Geometry check sheet. Reference: the model listing, model coordinates, mm. Face numbers are marked on the shaded views. A direction names the side the tool comes from. Coordinates: 2 decimals unless noted, no trailing zeros. Write each loop counter-clockwise with the first axis right and the second up, starting at its lowest first coordinate (ties: lowest second). Pieces come first, ordered by that corner, then holes. Notation, with made-up numbers: (-6.75, -15.75) -> (43.25, -15.75) arc R30 ccw to (43.25, 11.25) -> close; hole circle Ø11 at (-37, -39). An arc over 180 degrees is marked (long way). One line per question, with ' | ' between items.
from build123d import *

# Parameters (mm, degrees)
PAD_DEPTH           = 20
SKETCH002_W         = 100
SKETCH002_H         = 20
SKETCH002_W_2       = 96
SKETCH002_H_2       = 16
PAD001_DEPTH        = 6
SKETCH001_R         = 5
POCKET_DEPTH        = 2.5
LINEARPATTERN_COUNT = 6
LINEARPATTERN_PITCH = 14


with BuildPart() as part:
    # Sketch → Pad (new body)
    with BuildSketch(Plane.XY):
        Polygon((0, 100), (0, 27), (-4, 27), (-4, 15), (0, 15), (0, -3), (-2.5, -3), (-2.5, 0), (-97.5, 0), (-97.5, -3), (-100, -3), (-100, 2.5), (-56.035534, 2.5), (-2.5, 56.035534), (-2.5, 100), align=None)
        Polygon((-52.5, 2.5), (-2.5, 2.5), (-2.5, 12.5), (-6.5, 12.5), (-6.5, 29.5), (-2.5, 29.5), (-2.5, 52.5), align=None, mode=Mode.SUBTRACT)
    extrude(amount=PAD_DEPTH)

    # Sketch002 → Pad001 (join)
    with BuildSketch(Plane.XZ):
        with Locations((-50, 10)):
            Rectangle(SKETCH002_W, SKETCH002_H)
        with Locations((-50, 10)):
            Rectangle(SKETCH002_W_2, SKETCH002_H_2, mode=Mode.SUBTRACT)
    extrude(amount=-PAD001_DEPTH)

    # Sketch001 → Pocket (cut)
    with BuildSketch(Plane.XZ):
        with Locations((-89.5, 10)):
            Circle(SKETCH001_R)
    pocket = extrude(amount=-POCKET_DEPTH, mode=Mode.SUBTRACT)

    # LinearPattern: Pocket ×6
    with Locations(*[(i * LINEARPATTERN_PITCH, 0, 0) for i in range(1, LINEARPATTERN_COUNT)]):
        add(pocket, mode=Mode.SUBTRACT)


solid = part.part
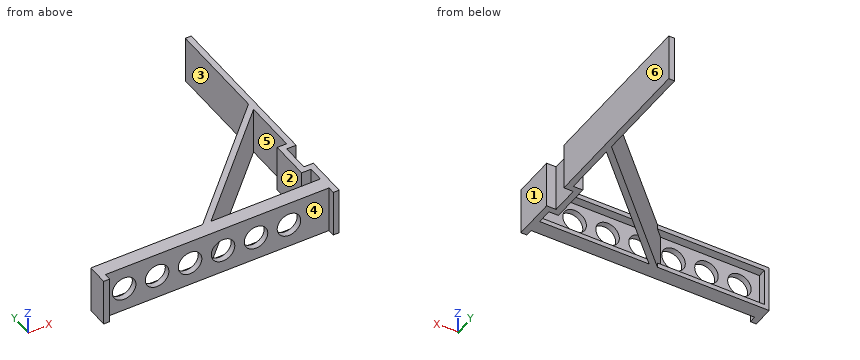
1. Cross-section at A-A on z = 3.25. Record the boundary of the cut face in (x, y).
Worked answers:
outline: (-100, -3) -> (-97.5, -3) -> (-97.5, 0) -> (-2.5, 0) -> (-2.5, -3) -> (0, -3) -> (0, 15) -> (-4, 15) -> (-4, 27) -> (0, 27) -> (0, 100) -> (-2.5, 100) -> (-2.5, 56.04) -> (-56.04, 2.5) -> (-98, 2.5) -> (-98, 6) -> (-100, 6) -> close; hole (-52.5, 2.5) -> (-2.5, 2.5) -> (-2.5, 12.5) -> (-6.5, 12.5) -> (-6.5, 29.5) -> (-2.5, 29.5) -> (-2.5, 52.5) -> close
2. Cross-section at B-B on x = -20.5. Record the boundary of the cut face in (y, z).
Worked answers:
outline: (0, 0) -> (6, 0) -> (6, 2) -> (2.5, 2) -> (2.5, 5.1) -> (0, 5.1) -> close; (0, 14.9) -> (2.5, 14.9) -> (2.5, 18) -> (6, 18) -> (6, 20) -> (0, 20) -> close; (34.5, 0) -> (38.04, 0) -> (38.04, 20) -> (34.5, 20) -> close
3. Go/stop test with flat-tipped pins: P1, Ø10, axis at y = 11.5, z = 17.5, coming from the -X side; P2, Ø1.2, axis at x = -4, z = 6.5, coming from the -Y side; P3, Ø5, axis at x = -19.5, z = 8, coming from the +Y side. Record where each tip stops, or that it passes through.
Worked answers:
P1: x = -52.04 | P2: y = 0 | P3: y = 41.54
4. Mould release check, pull along X, two halves, no side actions. Record for the marked faces 1, 2 and 3: released by +X, released by -X, zero draft, split by the parting line, or undercut.
Worked answers:
face 1: released by +X | face 2: undercut | face 3: released by -X
5. Cross-section at C-C on y = 46. Record the boundary of the cut face in (x, z).
Worked answers:
outline: (-12.54, 0) -> (-9, 0) -> (-9, 20) -> (-12.54, 20) -> close; (-2.5, 0) -> (0, 0) -> (0, 20) -> (-2.5, 20) -> close
6. Tool access check on the marked faces 4, 5 and 6. Record the directions out of +Z, -Z, +X, -X, +Y, -Y that give a thin tool (end or side, any length) a straight path to the whole face; none if there is none.
Worked answers:
face 4: +Z, -Z, -Y | face 5: +Z, -Z | face 6: +Z, -Z, +X, +Y, -Y
7. Material ranges on line 1 (X direction, y = 3, z = 4); line 2 (X direction, y = 93.5, z = 14.25); line 3 (Z direction, x = -19.5, y = 1.75), recorded low to high. Write a range as from..to.
Worked answers:
line 1: -100..-98, -55.54..-52, -2.5..0 | line 2: -2.5..0 | line 3: 0..5, 15..20
8. Cross-section at D-D on x = -61.5. Record the boundary of the cut face in (y, z).
Worked answers:
outline: (0, 0) -> (6, 0) -> (6, 2) -> (2.5, 2) -> (2.5, 5) -> (0, 5) -> close; (0, 15) -> (2.5, 15) -> (2.5, 18) -> (6, 18) -> (6, 20) -> (0, 20) -> close
